Could you check a few things on this model? Use its own coordinates, in mm. A direction names the side the tool comes from. Round coordinates to 2 decimals unless told otherwise and drop trailing zeros. Loops run counter-clockwise (first coordinate to the right, second up) from the corner with the lowest first, then second, coordinate; pieces in that order, holes last.
from build123d import *

# Parameters (mm, degrees)
F0_W     = 145
F0_H     = 86.6
F0_W_2   = 138.9
F0_H_2   = 80.5
F1_DEPTH = 31.15
F2_W     = 145
F2_H     = 86.6
F3_DEPTH = 3.05
F4_R     = 6.5
F5_DEPTH = 25
F6_R     = 1.5
F7_DEPTH = 25


with BuildPart() as f1:
    # F0 (on Front) → F1 (new body)
    with BuildSketch(Plane.XZ):
        Rectangle(F0_W, F0_H)
        Rectangle(F0_W_2, F0_H_2, mode=Mode.SUBTRACT)
    extrude(amount=F1_DEPTH)

    # F2 (on face) → F3 (join)
    with BuildSketch(Plane.XZ.offset(31.15)):
        Rectangle(F2_W, F2_H)
    extrude(amount=F3_DEPTH)

    # F4 (on face) → F5 (cut)
    with BuildSketch(Plane.XY.offset(43.3)):
        with Locations((-52.5, -15.2)):
            Circle(F4_R)
        with Locations((52.5, -15.2)):
            Circle(F4_R)
    extrude(amount=-F5_DEPTH, mode=Mode.SUBTRACT)

    # F6 (on face) → F7 (cut)
    with BuildSketch(Plane(origin=(0, 0, -43.3), x_dir=(1, 0, 0), z_dir=(0, 0, -1))):
        with Locations((-52.5, 15.2)):
            Circle(F6_R)
        with Locations((52.5, 15.2)):
            Circle(F6_R)
    extrude(amount=-F7_DEPTH, mode=Mode.SUBTRACT)


solid = f1.part
Item 1: Will these pins go through, and if not, where does the flat tip stop? pin 1 (4 mm diameter, centred on x = -29.5, z = -20.5, fed in from +Y); pin 2 (5 mm diameter, centred on x = 52.5, y = -15.2, fed in from +Z).
Results list:
pin 1: stops at y = -31.15
pin 2: stops at z = -40.25
Item 2: If we section it at B-B, the plane y = -2: Please give me the cut outline in (x, z), then the cut area to 3 significant figures.
Results list:
outline: (-72.5, -43.3) - (72.5, -43.3) - (72.5, 43.3) - (-72.5, 43.3) - close; hole (-69.45, -40.25) - (69.45, -40.25) - (69.45, 40.25) - (-69.45, 40.25) - close
area: 1,380 mm2
Item 3: If I drill on line 1 along X through (y, z) = (-15, -42); line 2 along Z through (x, y) = (-46.5, -11.5); line 3 along Y through (x, z) = (-52.5, -40.95), over which ranges is the centre line in solid material (lowest first)?
Results list:
line 1: x = -72.5 to -53.99, -51.01 to 51.01, 53.99 to 72.5
line 2: z = -43.3 to -40.25, 40.25 to 43.3
line 3: y = -34.2 to -16.7, -13.7 to 0
Item 4: We'd pull the mould along X, two halves only. Please class faces 4 (the flat face through (-72.5, -17, -1)), 5 (the cylindrical face through (51.654, -8.755, 41.796)), 6 (the flat face through (-1, -34.2, 1)): released by +X, released by -X, zero draft, split by the parting line, or undercut.
Results list:
face 4: released by -X
face 5: undercut
face 6: zero draft
Item 5: For faces 1 (the cylindrical face through (51.39, -16.21, -41.8)), 2 (the flat face through (-1, -15, 40.25)), 3 (the cylindrical face through (-53.346, -8.755, 41.796)), which set-ups out of +Z, -Z, +X, -X, +Y, -Y let a thin tool reach every point of the face, with its end or its side?
Results list:
face 1: +Z, -Z
face 2: +Y
face 3: +Z
Item 6: If we section it at A-A, the plane x = 52.5: Please give me the cut outline in (y, z), then the cut area to 3 significant figures.
Results list:
outline: (-34.2, -43.3) - (-16.7, -43.3) - (-16.7, -40.25) - (-31.15, -40.25) - (-31.15, 40.25) - (-21.7, 40.25) - (-21.7, 43.3) - (-34.2, 43.3) - close; (-13.7, -43.3) - (0, -43.3) - (0, -40.25) - (-13.7, -40.25) - close; (-8.7, 40.25) - (0, 40.25) - (0, 43.3) - (-8.7, 43.3) - close
area: 405 mm2
Item 7: If we section it at D-D, the plane x = -49: Please give me the cut outline in (y, z), then the cut area to 3 significant figures.
Results list:
outline: (-34.2, -43.3) - (0, -43.3) - (0, -40.25) - (-31.15, -40.25) - (-31.15, 40.25) - (-20.68, 40.25) - (-20.68, 43.3) - (-34.2, 43.3) - close; (-9.72, 40.25) - (0, 40.25) - (0, 43.3) - (-9.72, 43.3) - close
area: 421 mm2
Item 8: If we section it at C-C, the plane y = -15.2: Please give me the cut outline in (x, z), then the cut area to 3 significant figures.
Results list:
outline: (-72.5, -43.3) - (-54, -43.3) - (-54, -40.25) - (-69.45, -40.25) - (-69.45, 40.25) - (-59, 40.25) - (-59, 43.3) - (-72.5, 43.3) - close; (-51, -43.3) - (51, -43.3) - (51, -40.25) - (-51, -40.25) - close; (-46, 40.25) - (46, 40.25) - (46, 43.3) - (-46, 43.3) - close; (54, -43.3) - (72.5, -43.3) - (72.5, 43.3) - (59, 43.3) - (59, 40.25) - (69.45, 40.25) - (69.45, -40.25) - (54, -40.25) - close
area: 1,280 mm2
